from build123d import *

# Parameters (mm, degrees)
F4_R     = 4
F5_DEPTH = 45


# Not quite as in the source:
# - a feature names something its author has since deleted; it is built from what else it names


with BuildPart() as f1:
    # F0 (on Front) → F1 (revolve)
    with BuildSketch(Plane.XZ):
        with BuildLine():
            ThreePointArc((1.311079303, 6.2763909436), (-1.0236192616, 7.0769066725), (-3.4030299061, 6.4211263706))
            Line((-3.4030299061, 6.4211263706), (1.311079303, 6.2763909436))
        make_face()
        with BuildLine():
            Line((3.831038924, 6.1990216219), (8.6828378167, 6.0500587631))
            ThreePointArc((8.6828378167, 6.0500587631), (6.2786539333, 6.8318275323), (3.831038924, 6.1990216219))
        make_face()
        Polygon((-34.6867218614, 6.921078112), (-34.6867218614, 0), (10.3132781386, 0), (10.3132781386, 6), (8.6828378167, 6.0500587631), (3.831038924, 6.1990216219), (1.311079303, 6.2763909436), (-3.4030299061, 6.4211263706), (-19.6867218614, 6.921078112), align=None)
    revolve(axis=Axis((-12.1867218614, 0, 0), (1, 0, 0)))

    # F2 (on Front) → F3 (revolve)
    with BuildSketch(Plane.XZ):
        Polygon((-30.2853044122, -6.0204798356), (-30.2853044122, -6.921078112), (-30.2853044122, -10.421078112), (-28.2853044122, -10.421078112), (-28.2853044122, -6.921078112), (-28.2853044122, -6.0204798356), align=None)
        Polygon((-28.2853044122, 6.921078112), (-28.2853044122, 10.421078112), (-30.2853044122, 10.421078112), (-30.2853044122, 6.921078112), (-30.2853044122, 5.468968302), (-28.2853044122, 5.468968302), align=None)
    revolve(axis=Axis((-28.2853044122, 0, 8.671078112), (0, 0, -1)))

    # F4 (on face) → F5 (cut, through all)
    with BuildSketch(Plane(origin=(-34.6867218614, 0, 0), x_dir=(0, -1, 0), z_dir=(-1, 0, 0))):
        Circle(F4_R)
    extrude(amount=-F5_DEPTH, mode=Mode.SUBTRACT)


solid = f1.part
CAD build for the part. Positions are in the model's coordinates, mm. A direction names the side the tool comes from. Coordinates: 2 decimals unless noted, no trailing zeros. Write each loop counter-clockwise with the first axis right and the second up, starting at its lowest first coordinate (ties: lowest second). Pieces come first, ordered by that corner, then holes. Notation, with made-up numbers: M -5,46 L 20,46 A19 ccw 20,67 Z; hole C 58,67.5 d6. An arc over 180 degrees is marked long. Answer as a JSON object with one key per item and string values. Group by question number.
1) Wall check: line 1 (Z direction, x = 1.5, y = 0); line 2 (Z direction, x = -19.5, y = 0); line 3 (Y direction, x = -24.5, z = -3). Give the ranges that are in metal, low to high. Write a range as from..to.
2) Saw through at A-A (x = -29). Write the cut outline in (y, z).
3) Pin check, flat tips, straight feed: pin 1 Ø6 at (x, z) = (-10.5, 1) entering from +Y; pin 2 Ø3 at (x, z) = (1.5, -1) entering from -Y (3 decimals); pin 3 Ø2 at (x, z) = (-8.5, 6) entering from +Y. Stop position of each tip, or through.
4) Mould opens along Z. For faces 6 (the face through (-12.502, 0.867, -3.905)), 7 (the face through (10.313, 3.92, 1.42)), 8 (the face through (-27.29, -2.08, 6.6)), 9 (the face through (-28, 0, 10.421)) say: +Z half, -Z half, draft (parallel to the pull), parting line (faces both ways), or undercut.
5) Saw through at C-C (x = -13.5). Write the cut outline in (y, z), plus the area to 3 significant figures.
6) Saw through at B-B (x = -24). Write the cut outline in (y, z).
7) Tool access for faces 1 (the face through (9.67, -1.81, 5.74)), 2 (the face through (-28, 0, -10.421)), 3 (the face through (-28.025, 1.983, 8.497)), 4 (the face through (-26.287, 0.088, -8.55)), 5 (the face through (2.83, 6.08, -1.35)): list every direction of +Z, -Z, +X, -X, +Y, -Y with a clear straight run to the whole face (end or side of a thin tool).
Values follow:
{
 "1": {"line 1": "z = -6.27..-4, 4..6.27", "line 2": "z = -6.92..-4, 4..6.92", "line 3": "y = -6.24..-2.65, 2.65..6.24"},
 "2": {"outline": "M -1.87,-10.42 L 1.87,-10.42 L 1.87,-6.66 A6.92 ccw 1.87,6.66 L 1.87,10.42 L -1.87,10.42 L -1.87,6.66 A6.92 ccw -1.87,-6.66 Z; hole C 0,0 d8"},
 "3": {"pin 1": "stops at y = 6.73", "pin 2": "stops at y = -6.875", "pin 3": "stops at y = 4.27"},
 "4": {"face 6": "undercut", "face 7": "draft", "face 8": "parting line", "face 9": "+Z half"},
 "5": {"outline": "C 0,0 d13.46; hole C 0,0 d8", "area": "92.1 mm2"},
 "6": {"outline": "C 0,0 d13.84; hole C 0,0 d8"},
 "7": {"face 1": "+X", "face 2": "-Z, +X, -X, +Y, -Y", "face 3": "+Z", "face 4": "-Z", "face 5": "none"}
}
